Can you work these out from the model? Positions are in its coordinate system, mm. Coordinates: 2 decimals unless noted, no trailing zeros. Loops run counter-clockwise (first coordinate to the right, second up) from the corner with the lowest first, then second, coordinate; pieces in that order, holes last. Notation, with made-up numbers: M -11,1.25 L 8,1.25 A20 ccw 8,10.25 Z; hole C 56.25,-22 d5. An arc over 180 degrees is marked long. Return JSON: item names as keys, results as strings. Group by question number.
Autodesk Inventor part; units mm, degrees
ref_plane "YZ Plane" through (0, 0, 0) normal (1, 0, 0) x (0, 1, 0)
ref_plane "XZ Plane" through (0, 0, 0) normal (0, 1, 0) x (-1, 0, 0)
ref_plane "XY Plane" through (0, 0, 0) normal (0, 0, 1) x (1, 0, 0)
sketch "Sketch1" plane through (0, 0, 0) normal (0, 0, 1) x (1, 0, 0)
  circle A0 centre (0, 0) radius 1.5
  dimension "d0" = 3
extrude "Extrusion1" add sketch "Sketch1" along normal blind 30
sketch "Sketch4" plane through (0, 0, 30) normal (0, 0, 1) x (1, 0, 0)
  circle A0 centre (0, 0) radius 1.5
extrude "Extrusion3" add sketch "Sketch4" along normal blind 6.5
sketch "Sketch5" plane through (0, 0, 0) normal (0, 0, -1) x (-1, 0, 0)
  circle A0 centre (0, 0) radius 1.5
  circle A1 centre (0, 0) radius 1.5
extrude "Extrusion4" add sketch "Sketch5" along normal blind 6
properties part number "Extra Shaft"
1) Suppose I cut it at A-A, the plane z = 15.5. List the corners of the cut face in (x, y) for me, then the cut area to 3 significant figures.
2) Suppose I cut it at C-C, the plane y = -0.5. List the corners of the cut face in (x, z) for me, then the cut area to 3 significant figures.
3) If I drill on line 1 (Y direction, x = 0.1, z = 8.5); line 2 (X direction, y = -0.4, z = 22.5); line 3 (Y direction, x = -1.2, z = 23), over which ranges is the centre line in solid material (lowest first)? Write a range as from..to.
4) For pin 1 (1.5 mm diameter, centred on y = 1, z = 12.5, fed in from -X), with a flat end and sliding along its axis, tell me the tip position at first contact or that it passes through.
5) Suppose I cut it at B-B, the plane x = 1. List the corners of the cut face in (y, z) for me.
Returned:
{
 "1": {"outline": "C 0,0 d3", "area": "7.07 mm²"},
 "2": {"outline": "M -1.41,-6 L 1.41,-6 L 1.41,36.5 L -1.41,36.5 Z", "area": "120 mm²"},
 "3": {"line 1": "y = -1.5..1.5", "line 2": "x = -1.45..1.45", "line 3": "y = -0.9..0.9"},
 "4": {"pin 1": "stops at x = -1.48"},
 "5": {"outline": "M -1.12,-6 L 1.12,-6 L 1.12,36.5 L -1.12,36.5 Z"}
}
